Design review of the part built by this model. Coordinates are the model's own, in mm. Face numbers are marked on the shaded views. Coordinates: 2 decimals unless noted, no trailing zeros. Write each loop counter-clockwise with the first axis right and the second up, starting at its lowest first coordinate (ties: lowest second). Pieces come first, ordered by that corner, then holes.
Q1. Take a section at C-C, the plane x = 27. Write out the cut boundary in (y, z) (3 decimals), plus the area to 3 significant figures.
Q2. For L1, parallel to X at y = 35.5, z = 2.65; L2, parallel to Y at x = 31, z = 1.9; L3, parallel to Y at x = 23, z = 0.9, list the stretches that pass through material, from the lowest coordinate up.
Q3. Take a section at B-B, the plane y = 15. Write out the cut boundary in (x, z) (3 decimals).
Q4. The part is to be moulded in two halves that separate along Z. For the marked faces 1 and 2, say which applies: released by +Z, released by -Z, zero draft, split by the parting line, or undercut.
Q5. Take a section at A-A, the plane z = 0.95. Write out the cut boundary in (x, y), plus the area to 3 significant figures.
Autodesk Inventor part; units mm, degrees
ref_plane "YZ Plane" through (0, 0, 0) normal (1, 0, 0) x (0, 1, 0)
ref_plane "XZ Plane" through (0, 0, 0) normal (0, 1, 0) x (-1, 0, 0)
ref_plane "XY Plane" through (0, 0, 0) normal (0, 0, 1) x (1, 0, 0)
sketch "Sketch2" plane through (0, 0, 0) normal (0, 0, 1) x (1, 0, 0)
  line L0 (0, 0) -> (0, -55.88)
  line L1 (0, 0) -> (55.88, 0) construction
  line L2 (0, -55.88) -> (125.6284, -55.88)
  line L3 (125.6284, -55.88) -> (125.6284, 45.72)
  line L4 (125.6284, 45.72) -> (58.5724, 45.72)
  line L5 (58.5724, 45.72) -> (0, 0)
  dimension "d4" = 55.88
  dimension "d5" = 90
  dimension "d6" = 125.6284
  dimension "d7" = 101.6
  dimension "d8" = 90
  dimension "d9" = 67.056
  dimension "d10" = 90
extrude "Extrusion2" add sketch "Sketch2" along normal blind 3.175
properties part number "side plate" material "Aluminum 6061"
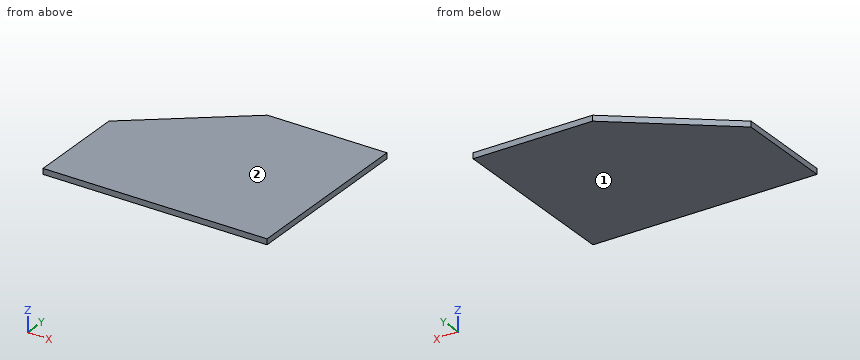
Responses:
1. outline: (-55.88, 0) - (21.075, 0) - (21.075, 3.175) - (-55.88, 3.175) - close
1. area: 244 mm2
2. L1: x = 45.48 to 125.63
2. L2: y = -55.88 to 24.2
2. L3: y = -55.88 to 17.95
3. outline: (19.217, 0) - (125.628, 0) - (125.628, 3.175) - (19.217, 3.175) - close
4. face 1: released by -Z
4. face 2: released by +Z
5. outline: (0, -55.88) - (125.63, -55.88) - (125.63, 45.72) - (58.57, 45.72) - (0, 0) - close
5. area: 11,400 mm2
